```python
from build123d import *

# Parameters (mm, degrees)
BOSS_EXTRUDE1_DEPTH = 135
SHELL1_T            = -2


with BuildPart() as part:
    # Sketch1 → Boss-Extrude1 (new, symmetric)
    with BuildSketch(Plane.XY):
        Polygon((550, 500), (-550, 500), (-550, 156), (-208, -612.144576675), (208, -612.144576675), (550, 156), align=None)
    extrude(amount=BOSS_EXTRUDE1_DEPTH, both=True)

    # Shell1
    shell1_openings = [part.faces().sort_by_distance(p)[0] for p in [
        (0, 25.973898383, -135),
    ]]
    offset(amount=SHELL1_T, openings=shell1_openings, kind=Kind.INTERSECTION)


solid = part.part
```
The model under review builds one solid part; all positions refer to its coordinate system, in mm. A direction names the side the tool comes from. Coordinates: 2 decimals unless noted, no trailing zeros. Write each loop counter-clockwise with the first axis right and the second up, starting at its lowest first coordinate (ties: lowest second). Pieces come first, ordered by that corner, then holes. Notation, with made-up numbers: (-13, 82) -> (27, 82) arc R14 ccw to (27, 95) -> close; hole circle Ø8 at (66.5, 22.5). An arc over 180 degrees is marked (long way). One line per item, written item: value. Start each with the question number.
Q1. Add section C-C, the plane x = 113. Give the boundary of the cut face in (y, z).
Q2. For faces 1 (the face through (376.606, -233.449, 1.89)), 2 (the face through (-8, 75, 133)), list the 3-axis set-ups (+Z, -Z, +X, -X, +Y, -Y) from which the entire face can be reached by the end or side of a thin tool; tool diameter is ignored.
Q3. Clearance check with flat-ended pins moving along their axes: P1, Ø4, axis at x = -5.5, y = -31.5, coming from the -Z side; P2, Ø10, axis at y = -194, z = -17, coming from the +X side; P3, Ø3, axis at y = -158.5, z = 69, coming from the +X side. State where each tip first meets the part, or that it passes through.
Q4. To check wall thickness, follow probe 1 along X at (y, z) = (373.5, -60); probe 2 along Y at (x, z) = (-139.5, 37); probe 3 along Y at (x, z) = (486, -77.5). State the ranges of each line that lie inside material, in increasing order.
Q5. Add section B-B, the plane y = 296. Give the boundary of the cut face in (x, z).
Q6. Add section A-A, the plane z = 29.5. Give the boundary of the cut face in (x, y), then the cut area to 3 significant figures.
Q7. The part is to be moulded in two halves that separate along Y. For faces 3 (the face through (374.96, -232.23, 0.88)), 4 (the face through (550, 326, 2)), 5 (the face through (-3, -612.145, 2)), say which applies: +Y half, -Y half, draft (parallel to the pull), parting line (faces both ways), or undercut.
Response:
1. outline: (-612.14, -135) -> (-610.14, -135) -> (-610.14, 133) -> (498, 133) -> (498, -135) -> (500, -135) -> (500, 135) -> (-612.14, 135) -> close
2. face 1: +Z, -Z, +X, -Y
2. face 2: -Z
3. P1: z = 133
3. P2: x = 396.4
3. P3: x = 410.64
4. probe 1: -550 to -548, 548 to 550
4. probe 2: -612.14 to -610.14, 498 to 500
4. probe 3: 12.25 to 17.17, 498 to 500
5. outline: (-550, -135) -> (-548, -135) -> (-548, 133) -> (548, 133) -> (548, -135) -> (550, -135) -> (550, 135) -> (-550, 135) -> close
6. outline: (-550, 156) -> (-208, -612.14) -> (208, -612.14) -> (550, 156) -> (550, 500) -> (-550, 500) -> close; hole (-548, 156.43) -> (-206.7, -610.14) -> (206.7, -610.14) -> (548, 156.43) -> (548, 498) -> (-548, 498) -> close
6. area: 7,760 mm²
7. face 3: undercut
7. face 4: draft
7. face 5: -Y half
